from build123d import *

# Parameters (mm, degrees)
BOSS_EXTRU_1_DEPTH = 50
CONG_1_R           = 0.75
ESQUISSE2_W        = 6
ESQUISSE2_H        = 5.312116381
ESQUISSE2_H_2      = 5.312116382
BOSS_EXTRU_2_DEPTH = 2
CONG_2_R           = 0.5


with BuildPart() as part:
    # Esquisse1 → Boss.-Extru.1 (new body)
    with BuildSketch(Plane.XY):
        Polygon((-4.120689655, 5.1), (-2.120689655, 5.1), (-2.120689655, 0), (-0.120689655, 0), (-0.120689655, 5.1), (1.879310345, 5.1), (1.879310345, -5.2), (-4.120689655, -5.2), align=None)
    extrude(amount=BOSS_EXTRU_1_DEPTH)

    # Congé1
    cong_1_edges = [part.edges().sort_by_distance(p)[0] for p in [
        (-4.120689655, 5.1, 25),
        (-2.120689655, 5.1, 25),
        (-0.120689655, 5.1, 25),
        (1.879310345, 5.1, 25),
    ]]
    fillet(cong_1_edges, radius=CONG_1_R)

    # Esquisse2 → Boss.-Extru.2 (add)
    with BuildSketch(Plane.XZ.offset(5.2)):
        with Locations((-7.120689655, 39.088656491)):
            Rectangle(ESQUISSE2_W, ESQUISSE2_H)
        with Locations((-7.100094061, 14.445055711)):
            Rectangle(ESQUISSE2_W, ESQUISSE2_H_2)
    extrude(amount=-BOSS_EXTRU_2_DEPTH)

    # Congé2
    cong_2_edges = [part.edges().sort_by_distance(p)[0] for p in [
        (-10.120689655, -3.2, 39.088656491),
        (-7.120689655, -3.2, 41.744714681),
        (-7.120689655, -3.2, 36.4325983),
        (-7.110391858, -3.2, 17.101113902),
        (-7.110391858, -3.2, 11.78899752),
        (-10.100094061, -3.2, 14.445055711),
    ]]
    fillet(cong_2_edges, radius=CONG_2_R)


solid = part.part
Source: CAD feature listing. Evaluate the final solid. Frame: model axes, mm. A direction names the side the tool comes from. Round coordinates to 2 decimals unless told otherwise and drop trailing zeros. Write each loop counter-clockwise with the first axis right and the second up, starting at its lowest first coordinate (ties: lowest second). Pieces come first, ordered by that corner, then holes. Notation, with made-up numbers: M -18,43.5 L 30,43.5 A19 ccw 30,57.5 Z; hole C 2.5,42 d7. An arc over 180 degrees is marked long. One line per item, written item: value. Start each with the question number.
Item 1: Ray query, L1, parallel to X at y = 2, z = 17; L2, parallel to Y at x = -5, z = 40.5; L3, parallel to Y at x = 1.25, z = 34. Return the intervals inside material, ascending. Write a range as from..to.
Item 2: Section query B-B (x = -7.5). Return the cut outline in (y, z).
Item 3: Section query A-A (y = 1.5). Return the cut outline in (x, z), plus the area to 3 significant figures.
Item 4: Section query D-D (y = -2.5). Return the cut outline in (x, z), plus the area to 3 significant figures.
Item 5: Section query C-C (z = 28.5). Return the cut outline in (x, y), plus the area to 3 significant figures.
Item 6: Mould query, pull axis Z, two halves, no side actions, for faces 1 (the flat face through (-1, -1, 50)), 2 (the flat face through (-7, -4, 17.101)), 3 (the flat face through (-7, -4, 36.433)), 4 (the flat face through (-10.121, -4, 39)). Classes: pulls with the +Z half, pulls with the -Z half, needs draft (parallel to the pull), parting line crosses it, or undercut.
Item 7: Pin query (flat end, axial travel): pin 1 (1.2 mm diameter, centred on x = -6, y = -4, fed in from +Z); pin 2 (1 mm diameter, centred on y = -3, z = 18.5, fed in from -X); pin 3 (1.6 mm diameter, centred on x = -7.5, y = -4.5, fed in from -Z). Return the tip coordinate at first contact, or that it passes through.
Item 8: Set-up query: faces 5 (the flat face through (-7, -4, 11.789)), 6 (the flat face through (-0.121, 2, 25)), 7 (the flat face through (-4.121, 0, 25)), 8 (the flat face through (-7, -3.2, 14)). Return all of +Z, -Z, +X, -X, +Y, -Y with unobstructed straight access to the full face (end or side cutting, diameter ignored); none if empty.
Result set:
1. L1: x = -4.12..-2.12, -0.12..1.88
1. L2: y = -5.2..-3.2
1. L3: y = -5.2..5.09
2. outline: M -5.2,11.79 L -3.7,11.79 A0.5 ccw -3.2,12.29 L -3.2,16.6 A0.5 ccw -3.7,17.1 L -5.2,17.1 Z; M -5.2,36.43 L -3.7,36.43 A0.5 ccw -3.2,36.93 L -3.2,41.24 A0.5 ccw -3.7,41.74 L -5.2,41.74 Z
3. outline: M -4.12,0 L -2.12,0 L -2.12,50 L -4.12,50 Z; M -0.12,0 L 1.88,0 L 1.88,50 L -0.12,50 Z
3. area: 200 mm²
4. outline: M -4.12,0 L 1.88,0 L 1.88,50 L -4.12,50 Z
4. area: 300 mm²
5. outline: M -4.12,-5.2 L 1.88,-5.2 L 1.88,4.35 A0.75 ccw 1.13,5.1 L 0.63,5.1 A0.75 ccw -0.12,4.35 L -0.12,0 L -2.12,0 L -2.12,4.35 A0.75 ccw -2.87,5.1 L -3.37,5.1 A0.75 ccw -4.12,4.35 Z
5. area: 51.1 mm²
6. face 1: pulls with the +Z half
6. face 2: undercut
6. face 3: undercut
6. face 4: needs draft
7. pin 1: stops at z = 41.74
7. pin 2: stops at x = -4.12
7. pin 3: stops at z = 11.79
8. face 5: -Z, -X, +Y, -Y
8. face 6: +Z, -Z, +Y
8. face 7: -X, +Y
8. face 8: +Z, -Z, -X, +Y
